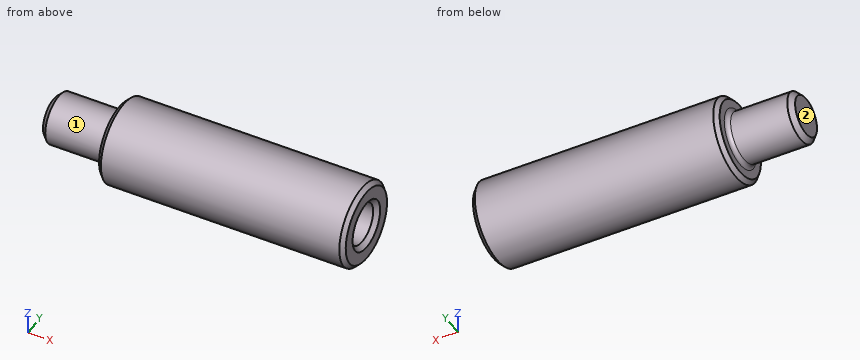
from build123d import *


with BuildPart() as part:
    # Sketch1 → Revolve1 (revolve)
    with BuildSketch(Plane.XY, mode=Mode.PRIVATE) as revolve1_sk:
        Polygon((0, 0), (0, 4.5), (0.5, 5), (29.5, 5), (30, 4.5), (30, 0), align=None)
    revolve(revolve1_sk.sketch.rotate(Axis((30, 0, 0), (-1, 0, 0)), 270), axis=Axis((30, 0, 0), (-1, 0, 0)))

    # Sketch2 → Revolve2 (revolve)
    with BuildSketch(Plane.XY, mode=Mode.PRIVATE) as revolve2_sk:
        with BuildLine():
            Line((-8, 0), (-8, 2.3865))
            Line((-8, 2.3865), (-7.3865, 3))
            Line((-7.3865, 3), (-0.5, 3))
            ThreePointArc((-0.5, 3), (-0.146446609, 3.146446609), (0, 3.5))
            Line((0, 3.5), (0, 0))
            Line((0, 0), (-8, 0))
        make_face()
    revolve(revolve2_sk.sketch.rotate(Axis((0, 0, 0), (-1, 0, 0)), 270), axis=Axis((0, 0, 0), (-1, 0, 0)))

    # Sketch3 → Cut-Revolve1 (revolve, cut)
    with BuildSketch(Plane.XY, mode=Mode.PRIVATE) as cut_revolve1_sk:
        Polygon((5, 0), (6.419415637, 2.4585), (29.4585, 2.4585), (30, 3), (30, 0), align=None)
    revolve(cut_revolve1_sk.sketch.rotate(Axis((30, 0, 0), (-1, 0, 0)), 270), axis=Axis((30, 0, 0), (-1, 0, 0)), mode=Mode.SUBTRACT)


solid = part.part
Geometry check sheet. Reference: the model listing, model coordinates, mm. Face numbers are marked on the shaded views. A direction names the side the tool comes from. Give positions to 0.01 mm unless a question says otherwise; leave off trailing zeros. Order: outer loops, then holes, each group sorted by start corner. A loop starts at its lowest first (then second) coordinate and runs counter-clockwise, first axis right, second up.
1. Scan lines: line 1 (Y direction, x = 20, z = 0); line 2 (Z direction, x = 27, y = -1); line 3 (X direction, y = -1.5, z = 3.25). Record each from-to range of solid material in increasing order.
Completed:
line 1: y = -5 to -2.46, 2.46 to 5
line 2: z = -4.9 to -2.25, 2.25 to 4.9
line 3: x = 0 to 30
2. Sectioned sample at B-B (x = -3). Record the boundary of the cut face in (y, z), then the cut area to 3 significant figures.
Completed:
outline: circle Ø6 at (0, 0)
area: 28.3 mm2
3. Sectioned sample at A-A (x = 19). Record the boundary of the cut face in (y, z).
Completed:
outline: circle Ø10 at (0, 0); hole circle Ø4.92 at (0, 0)
4. Depth check by flat-ended pin: pin 1 (1.5 mm diameter, centred on x = -0.5, y = 0.5, fed in from -Z); pin 2 (1 mm diameter, centred on x = 0.5, z = 1, fed in from +Y); pin 3 (3 mm diameter, centred on y = 0, z = 0, fed in from +X). Enter the tip coordinate at first touch or a pass-through.
Completed:
pin 1: stops at z = -4.73
pin 2: stops at y = 4.97
pin 3: stops at x = 5.87
5. Access from +Z, -Z, +X, -X, +Y, -Y to the whole of each face (thin tool, end or side, straight path). Record for the marked faces 1 and 2.
Completed:
face 1: -X
face 2: +Z, -Z, -X, +Y, -Y
